```python
from build123d import *

# Parameters (mm, degrees)
F0_W      = 63
F0_H      = 46
F1_DEPTH  = 26.3
F3_DEPTH  = 21.3
F4_R      = 2.15
F5_DEPTH  = 5.001
F6_W      = 12.75
F6_H      = 8.25
F7_DEPTH  = 63.001
F8_W      = 38
F8_H      = 46
F9_DEPTH  = 26.3
F10_R     = 3.75
F11_DEPTH = 2.6


with BuildPart() as f1:
    # F0 (on Top) → F1 (new body)
    with BuildSketch(Plane.XY):
        with Locations((31.5, 23)):
            Rectangle(F0_W, F0_H)
    extrude(amount=F1_DEPTH)

    # F2 (on face) → F3 (cut)
    with BuildSketch(Plane.XY.offset(26.3)):
        with BuildLine():
            Line((7, 28), (0, 28))
            Line((0, 28), (0, 18))
            Line((0, 18), (7, 18))
            ThreePointArc((7, 18), (12, 23), (7, 28))
        make_face()
        with BuildLine():
            Line((63, 18), (63, 28))
            Line((63, 28), (56, 28))
            ThreePointArc((56, 28), (51, 23), (56, 18))
            Line((56, 18), (63, 18))
        make_face()
    extrude(amount=-F3_DEPTH, mode=Mode.SUBTRACT)

    # F4 (on face) → F5 (cut, through all)
    with BuildSketch(Plane.XY.offset(5)):
        with BuildLine():
            Line((8.9, 25.15), (6.1, 25.15))
            ThreePointArc((6.1, 25.15), (3.95, 23), (6.1, 20.85))
            Line((6.1, 20.85), (8.9, 20.85))
            ThreePointArc((8.9, 20.85), (11.05, 23), (8.9, 25.15))
        make_face()
        with Locations((55.45, 23)):
            Circle(F4_R)
    extrude(amount=-F5_DEPTH, mode=Mode.SUBTRACT)

    # F6 (on face) → F7 (cut, through all)
    with BuildSketch(Plane.YZ.offset(63)):
        with Locations((37.275, 19.575)):
            Rectangle(F6_W, F6_H)
        with Locations((8.725, 19.575)):
            Rectangle(F6_W, F6_H)
    extrude(amount=-F7_DEPTH, mode=Mode.SUBTRACT)

    # F8 (on Top) → F9 (join, through all)
    with BuildSketch(Plane.XY):
        with Locations((31.5, 23)):
            Rectangle(F8_W, F8_H)
    extrude(amount=F9_DEPTH)

    # F10 (on face) → F11 (cut, through all)
    with BuildSketch(Plane.XY.offset(26.3)):
        with Locations((6, 38)):
            Circle(F10_R)
        with Locations((6, 8)):
            Circle(F10_R)
        with Locations((57, 38)):
            Circle(F10_R)
        with Locations((57, 8)):
            Circle(F10_R)
    extrude(amount=-F11_DEPTH, mode=Mode.SUBTRACT)


solid = f1.part
```
Check sheet for the modelled part. Datum: model origin and axes. Units: mm. A direction names the side the tool comes from. Round coordinates to 2 decimals unless told otherwise and drop trailing zeros. Write each loop counter-clockwise with the first axis right and the second up, starting at its lowest first coordinate (ties: lowest second). Pieces come first, ordered by that corner, then holes. Notation, with made-up numbers: (32, 36) -> (42, 36) arc R20 ccw to (42, 40) -> close; hole circle Ø11 at (-16, 63). An arc over 180 degrees is marked (long way). Put each result on its own line as item: value.
(1) Sectioned sample at A-A (y = 8). Enter the section's corners in (x, z), plus the area to 3 significant figures.
Values found:
outline: (0, 0) -> (63, 0) -> (63, 15.45) -> (50.5, 15.45) -> (50.5, 23.7) -> (53.25, 23.7) -> (53.25, 26.3) -> (9.75, 26.3) -> (9.75, 23.7) -> (12.5, 23.7) -> (12.5, 15.45) -> (0, 15.45) -> close; (0, 23.7) -> (2.25, 23.7) -> (2.25, 26.3) -> (0, 26.3) -> close; (60.75, 23.7) -> (63, 23.7) -> (63, 26.3) -> (60.75, 26.3) -> close
area: 1,410 mm^2
(2) Tool access check on faces 1 (the face through (59, 18, 16)), 2 (the face through (6, 15.1, 20)), 3 (the face through (3, 23, 5)), 4 (the face through (57, 43.65, 20)), 5 (the face through (60.464, 36.564, 25.018)). Record the directions out of +Z, -Z, +X, -X, +Y, -Y that give a thin tool (end or side, any length) a straight path to the whole face; none if there is none.
Values found:
face 1: +Z, +X
face 2: -X
face 3: +Z, -X
face 4: +X
face 5: +Z
(3) Material ranges on line 1 (Y direction, x = 6, z = 25.7); line 2 (Y direction, x = 60.5, z = 17.25); line 3 (Z direction, x = 12, y = 8), recorded low to high.
Values found:
line 1: y = 0 to 4.25, 11.75 to 18, 28 to 34.25, 41.75 to 46
line 2: y = 0 to 2.35, 15.1 to 18, 28 to 30.9, 43.65 to 46
line 3: z = 0 to 15.45, 23.7 to 26.3
(4) Go/stop test with flat-tipped pins: pin 1 Ø7 at (x, y) = (6, 8) entering from -Z; pin 2 Ø2.5 at (y, z) = (10.5, 18.5) entering from -X; pin 3 Ø4 at (y, z) = (34, 20) entering from +X. Record where each tip stops, or that it passes through.
Values found:
pin 1: stops at z = 0
pin 2: stops at x = 12.5
pin 3: stops at x = 50.5
(5) Sectioned sample at C-C (y = 23). Enter the section's corners in (x, z).
Values found:
outline: (0, 0) -> (3.95, 0) -> (3.95, 5) -> (0, 5) -> close; (11.05, 0) -> (53.3, 0) -> (53.3, 5) -> (51, 5) -> (51, 26.3) -> (12, 26.3) -> (12, 5) -> (11.05, 5) -> close; (57.6, 0) -> (63, 0) -> (63, 5) -> (57.6, 5) -> close
(6) Mould release check, pull along Y, two halves, no side actions. Record for faces 6 (the face through (31, 23, 26.3)), 7 (the face through (57, 2.35, 20)), 8 (the face through (31, 46, 13)), 9 (the face through (50.5, 37, 20)): released by +Y, released by -Y, zero draft, split by the parting line, or undercut.
Values found:
face 6: zero draft
face 7: undercut
face 8: released by +Y
face 9: undercut
(7) Sectioned sample at B-B (z = 22.25). Enter the section's corners in (x, y).
Values found:
outline: (0, 0) -> (63, 0) -> (63, 2.35) -> (50.5, 2.35) -> (50.5, 15.1) -> (63, 15.1) -> (63, 18) -> (56, 18) arc R5 cw to (56, 28) -> (63, 28) -> (63, 30.9) -> (50.5, 30.9) -> (50.5, 43.65) -> (63, 43.65) -> (63, 46) -> (0, 46) -> (0, 43.65) -> (12.5, 43.65) -> (12.5, 30.9) -> (0, 30.9) -> (0, 28) -> (7, 28) arc R5 cw to (7, 18) -> (0, 18) -> (0, 15.1) -> (12.5, 15.1) -> (12.5, 2.35) -> (0, 2.35) -> close
(8) Sectioned sample at D-D (z = 8). Enter the section's corners in (x, y).
Values found:
outline: (0, 0) -> (63, 0) -> (63, 18) -> (56, 18) arc R5 cw to (56, 28) -> (63, 28) -> (63, 46) -> (0, 46) -> (0, 28) -> (7, 28) arc R5 cw to (7, 18) -> (0, 18) -> close
